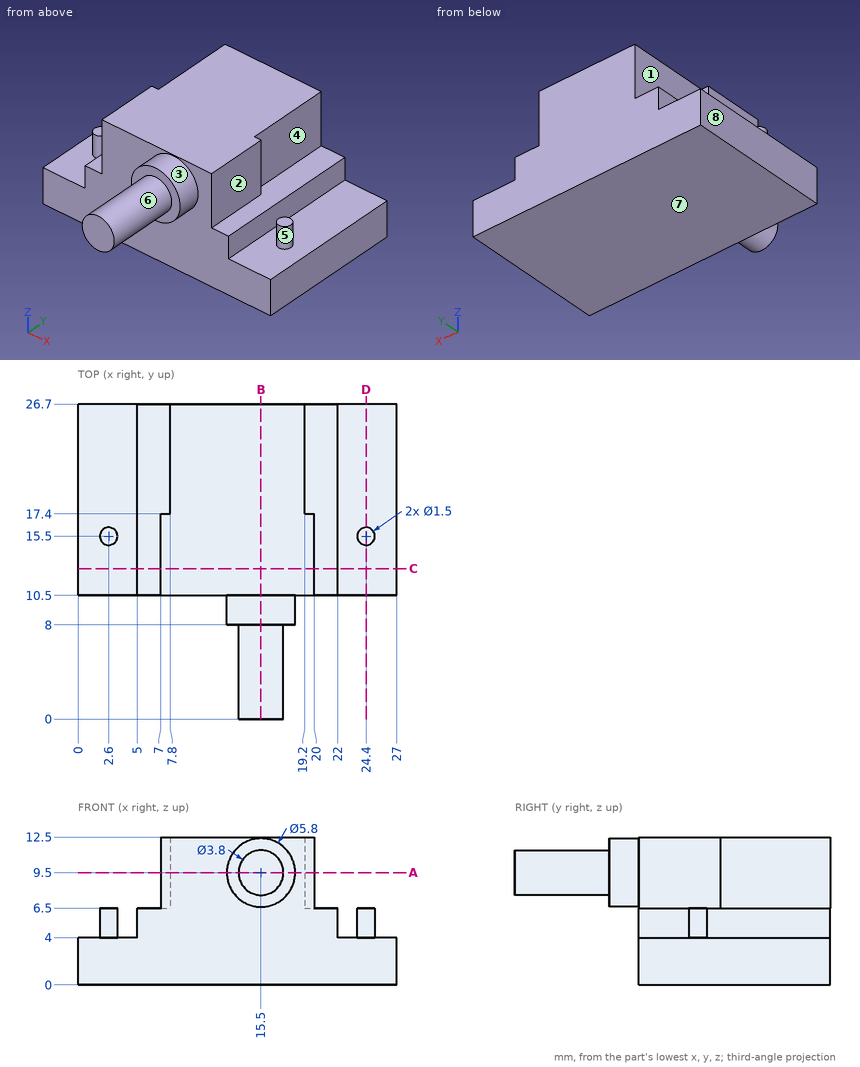
Answer from the drawing. Dimensions are ordinates in mm from the lowest x, y and z of the part. A direction names the side the tool comes from. Coordinates: 2 decimals unless noted, no trailing zeros. Loops run counter-clockwise (first coordinate to the right, second up) from the corner with the lowest first, then second, coordinate; pieces in that order, holes last.
1) Flat-ended cylindrical pins translate along their axes: pin 1 (2 mm diameter, centred on x = 4.5, z = 8, fed in from -Y); pin 2 (1.8 mm diameter, centred on y = 22, z = 11, fed in from -X); pin 3 (2 mm diameter, centred on y = 15, z = 5.5, fed in from +X); pin 4 (5.5 mm diameter, centred on x = 25.5, y = 22, fed in from +Z). Find the tip coordinate at first contact, or state that the pin passes through.
Results:
pin 1: passes through
pin 2: stops at x = 7.8
pin 3: stops at x = 25.15
pin 4: stops at z = 4
2) Section D-D (x = 24.4) is taken. Give the vertices of the cut face in (y, z), plus the area to 4 significant figures.
Results:
outline: (10.5, 0) - (26.7, 0) - (26.7, 4) - (16.25, 4) - (16.25, 6.5) - (14.75, 6.5) - (14.75, 4) - (10.5, 4) - close
area: 68.55 mm2
3) Section B-B (x = 15.5) is taken. Give the vertices of the cut face in (y, z), plus the area to 3 significant figures.
Results:
outline: (0, 7.6) - (8, 7.6) - (8, 6.6) - (10.5, 6.6) - (10.5, 0) - (26.7, 0) - (26.7, 12.5) - (10.5, 12.5) - (10.5, 12.4) - (8, 12.4) - (8, 11.4) - (0, 11.4) - close
area: 247 mm2
4) For a pull along X with two mould halves and no side action, classify the marked faces 5, 6, 7 and 8 as +X half, -X half, draft (parallel to the pull), parting line (faces both ways), or undercut.
Results:
face 5: undercut
face 6: parting line
face 7: draft
face 8: -X half
5) Section C-C (y = 12.75) is taken. Give the vertices of the cut face in (x, z).
Results:
outline: (0, 0) - (27, 0) - (27, 4) - (22, 4) - (22, 6.5) - (20, 6.5) - (20, 12.5) - (7, 12.5) - (7, 6.5) - (5, 6.5) - (5, 4) - (0, 4) - close
6) For the marked faces 1, 2, 3 and 4, determine the directions among +Z, -Z, +X, -X, +Y, -Y from which every point of the face is accessible in a straight line to the end or side of a thin tool.
Results:
face 1: +Z, -X, +Y
face 2: +Z, +X, +Y, -Y
face 3: -Y
face 4: +Z, +X, +Y
7) Consider probe 1 along X at (y, z) = (16.75, 10); probe 2 along X at (y, z) = (19.25, 7); probe 3 along Y at (x, z) = (11, 10). Determine where each line is inside the solid, lowest interval first.
Results:
probe 1: x = 7 to 20
probe 2: x = 7.8 to 19.2
probe 3: y = 10.5 to 26.7
8) Section A-A (z = 9.5) is taken. Give the vertices of the cut face in (x, y), plus the area to 3 significant figures.
Results:
outline: (7, 10.5) - (12.6, 10.5) - (12.6, 8) - (13.6, 8) - (13.6, 0) - (17.4, 0) - (17.4, 8) - (18.4, 8) - (18.4, 10.5) - (20, 10.5) - (20, 17.4) - (19.2, 17.4) - (19.2, 26.7) - (7.8, 26.7) - (7.8, 17.4) - (7, 17.4) - close
area: 241 mm2
